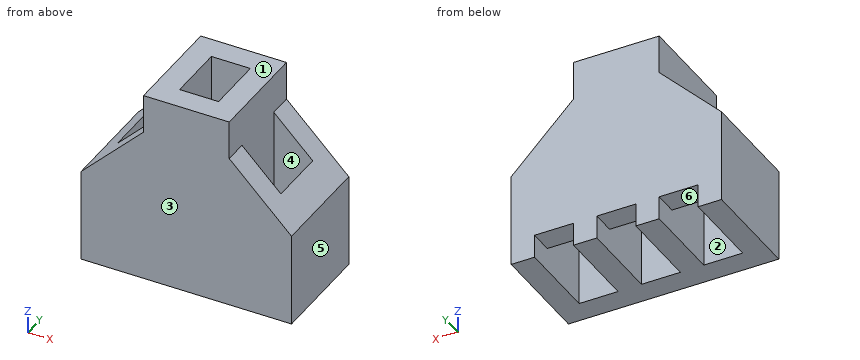
from build123d import *

# Parameters (mm, degrees)
F0_W     = 5
F0_H     = 7.5
F1_DEPTH = 25
F2_DEPTH = 20
F4_DEPTH = 25
F5_W     = 5
F5_H     = 3
F6_DEPTH = 25


with BuildPart() as f1:
    # F0 (on Top) → F1 (new body)
    with BuildSketch(Plane.XY):
        Polygon((5.5, 6.75), (-5.5, 6.75), (-5.5, 3.75), (-5.5, -3.75), (-5.5, -6.75), (5.5, -6.75), (5.5, -3.75), (5.5, 3.75), align=None)
        Rectangle(F0_W, F0_H, mode=Mode.SUBTRACT)
    extrude(amount=F1_DEPTH)

    # F0 (on Top) → F2 (join)
    with BuildSketch(Plane.XY):
        Polygon((-5.5, 3.75), (-5.5, 6.75), (-13.5, 6.75), (-13.5, -6.75), (-5.5, -6.75), (-5.5, -3.75), (-10.5, -3.75), (-10.5, 3.75), align=None)
        Polygon((13.5, 6.75), (5.5, 6.75), (5.5, 3.75), (10.5, 3.75), (10.5, -3.75), (5.5, -3.75), (5.5, -6.75), (13.5, -6.75), align=None)
    extrude(amount=F2_DEPTH)

    # F3 (on face) → F4 (cut)
    with BuildSketch(Plane.XZ.offset(6.75)):
        Polygon((-13.5, 12), (-5.5, 20), (-13.5, 20), align=None)
        Polygon((13.5, 20), (5.5, 20), (13.5, 12), align=None)
    extrude(amount=-F4_DEPTH, mode=Mode.SUBTRACT)

    # F5 (on Front) → F6 (cut)
    with BuildSketch(Plane.XZ):
        with Locations((-8, 1.5)):
            Rectangle(F5_W, F5_H)
        with Locations((0, 1.5)):
            Rectangle(F5_W, F5_H)
        with Locations((8, 1.5)):
            Rectangle(F5_W, F5_H)
    extrude(amount=-F6_DEPTH, mode=Mode.SUBTRACT)


solid = f1.part
Source: CAD feature listing. Evaluate the final solid. Frame: model axes, mm. Face numbers are marked on the shaded views. A direction names the side the tool comes from. Round coordinates to 2 decimals unless told otherwise and drop trailing zeros. Loops run counter-clockwise (first coordinate to the right, second up) from the corner with the lowest first, then second, coordinate; pieces in that order, holes last. Notation, with made-up numbers: (-26.75, -12) - (-18.75, -12) arc R24 ccw to (-18.75, 21) - close; hole circle Ø4 at (-16, 24). An arc over 180 degrees is marked (long way). Write item = value, one per line. Start each with the question number.
Item 1: Material intervals for line 1 (X direction, y = 2.25, z = 1.5); line 2 (Y direction, x = 1.25, z = 9); line 3 (X direction, y = 0.75, z = 21.5), sorted ascending.
Item 2: Mould query, pull axis Y, two halves, no side actions, for the marked faces 1, 2 and 3. Classes: released by +Y, released by -Y, zero draft, split by the parting line, or undercut.
Item 3: Section query A-A on x = -7.25. Output: boundary loops of the cut face in (y, z), plus the area to 4 significant figures.
Item 4: Section query B-B on z = 6. Output: boundary loops of the cut face in (x, y), plus the area to 3 significant figures.
Item 5: Reachability of the marked faces 4, 5 and 6 from +Z, -Z, +X, -X, +Y, -Y: full face, straight path, thin tool, end or side. Return the list, or none.
Item 6: Section query C-C on z = 17.5. Output: boundary loops of the cut face in (x, y), plus the area to 3 significant figures.
Item 7: First-contact query: pin 1 Ø3.5 at (x, y) = (-0.5, 6) entering from -Z; pin 2 Ø5 at (y, z) = (2.5, 16.5) entering from +X. Flat tips, straight axial feed; report the tip coordinate or a pass-through.
Item 8: Section query D-D on y = 2.5. Output: boundary loops of the cut face in (x, z).
Results list:
q1.line_1 = -13.5 to -10.5, -5.5 to -2.5, 2.5 to 5.5, 10.5 to 13.5
q1.line_2 = -6.75 to -3.75, 3.75 to 6.75
q1.line_3 = -5.5 to -2.5, 2.5 to 5.5
q2.face_1 = zero draft
q2.face_2 = undercut
q2.face_3 = released by -Y
q3.outline = (-6.75, 0) - (-3.75, 0) - (-3.75, 18.25) - (-6.75, 18.25) - close; (3.75, 3) - (6.75, 3) - (6.75, 18.25) - (3.75, 18.25) - close
q3.area = 100.5 mm²
q4.outline = (-13.5, -6.75) - (13.5, -6.75) - (13.5, 6.75) - (-13.5, 6.75) - close; hole (-10.5, -3.75) - (-5.5, -3.75) - (-5.5, 3.75) - (-10.5, 3.75) - close; hole (-2.5, -3.75) - (2.5, -3.75) - (2.5, 3.75) - (-2.5, 3.75) - close; hole (5.5, -3.75) - (10.5, -3.75) - (10.5, 3.75) - (5.5, 3.75) - close
q4.area = 252 mm²
q5.face_4 = +Z, -Z
q5.face_5 = +Z, -Z, +X, +Y, -Y
q5.face_6 = -Z, +Y
q6.outline = (-8, -6.75) - (8, -6.75) - (8, -3.75) - (5.5, -3.75) - (5.5, 3.75) - (8, 3.75) - (8, 6.75) - (-8, 6.75) - (-8, 3.75) - (-5.5, 3.75) - (-5.5, -3.75) - (-8, -3.75) - close; hole (-2.5, -3.75) - (2.5, -3.75) - (2.5, 3.75) - (-2.5, 3.75) - close
q6.area = 141 mm²
q7.pin_1 = 3
q7.pin_2 = 11.5
q8.outline = (-13.5, 0) - (-10.5, 0) - (-10.5, 15) - (-13.5, 12) - close; (-5.5, 0) - (-2.5, 0) - (-2.5, 25) - (-5.5, 25) - close; (2.5, 0) - (5.5, 0) - (5.5, 25) - (2.5, 25) - close; (10.5, 0) - (13.5, 0) - (13.5, 12) - (10.5, 15) - close
